from build123d import *

# Parameters (mm, degrees)
F0_W      = 40
F0_H      = 28
F1_DEPTH  = 1.5
F3_R      = 1.5
F4_DEPTH  = 1.501
F5_R      = 1.15
F6_DEPTH  = 1.501
F7_W      = 1.5
F7_H      = 28
F8_DEPTH  = 8
F9_R      = 3
F10_DEPTH = 1.501


with BuildPart() as f1:
    # F0 (on Front) → F1 (new body)
    with BuildSketch(Plane.XZ):
        with Locations((20, -14)):
            Rectangle(F0_W, F0_H)
    extrude(amount=F1_DEPTH)

    # F3 (on face) → F4 (cut, through all)
    with BuildSketch(Plane(origin=(0, 0, 0), x_dir=(-1, 0, 0), z_dir=(0, 1, 0))):
        with Locations((-38, -26)):
            Circle(F3_R)
        with Locations((-9, -24)):
            Circle(F3_R)
        with Locations((-9, -4)):
            Circle(F3_R)
    extrude(amount=-F4_DEPTH, mode=Mode.SUBTRACT)

    # F5 (on face) → F6 (cut, through all)
    with BuildSketch(Plane(origin=(0, 0, 0), x_dir=(-1, 0, 0), z_dir=(0, 1, 0))):
        with Locations((-20.5, -24)):
            Circle(F5_R)
        with Locations((-30.490284, -23.559283)):
            Circle(F5_R)
    extrude(amount=-F6_DEPTH, mode=Mode.SUBTRACT)

    # F7 (on face) → F8 (join)
    with BuildSketch(Plane.YZ.offset(40)):
        with Locations((-0.75, -14)):
            Rectangle(F7_W, F7_H)
    extrude(amount=F8_DEPTH)

    # F9 (on face) → F10 (cut, through all)
    with BuildSketch(Plane(origin=(0, 0, 0), x_dir=(-1, 0, 0), z_dir=(0, 1, 0))):
        with Locations((-38, -10)):
            Circle(F9_R)
    extrude(amount=-F10_DEPTH, mode=Mode.SUBTRACT)


solid = f1.part
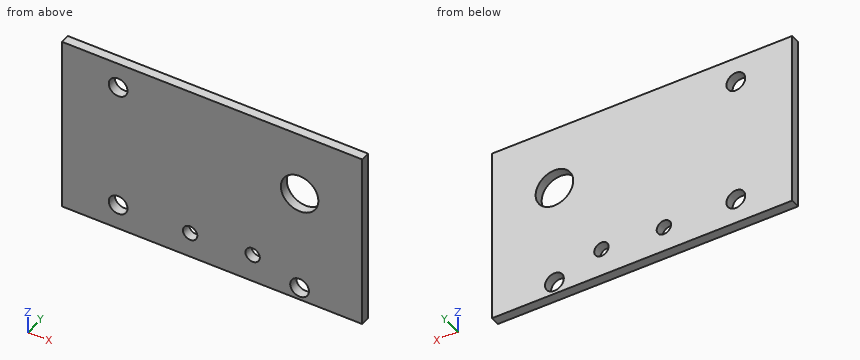
The model under review builds one solid part; all positions refer to its coordinate system, in mm. Round coordinates to 2 decimals unless told otherwise and drop trailing zeros. Loops run counter-clockwise (first coordinate to the right, second up) from the corner with the lowest first, then second, coordinate; pieces in that order, holes last. Notation, with made-up numbers: M 86,71 L 103,71 A20 cw 103,101 Z; hole C 88.5,-7 d8. An arc over 180 degrees is marked long. Answer as a JSON object with one key per item and string values.
Item 1: We need section B-B, the plane z = -10. State the section outline as (x, y) points, and give its area (3 significant figures).
Check sheet entries:
{"outline": "M 0,-1.5 L 35,-1.5 L 35,0 L 0,0 Z; M 41,-1.5 L 48,-1.5 L 48,0 L 41,0 Z", "area": "63.0 mm2"}
Item 2: We need section C-C, the plane x = 38. State the section outline as (y, z) points, and give its area (3 significant figures).
Check sheet entries:
{"outline": "M -1.5,-28 L 0,-28 L 0,-27.5 L -1.5,-27.5 Z; M -1.5,-24.5 L 0,-24.5 L 0,-13 L -1.5,-13 Z; M -1.5,-7 L 0,-7 L 0,0 L -1.5,0 Z", "area": "28.5 mm2"}
Item 3: Clearance check with flat-ended pins moving along their axes: P1, Ø2.5, axis at x = 9, z = -24, coming from the +Y side; P2, Ø5, axis at x = 30, z = -22.5, coming from the +Y side. State where each tip first meets the part, or that it passes through.
Check sheet entries:
{"P1": "through", "P2": "y = 0"}
Item 4: We need section D-D, the plane y = -1.1. State the section outline as (x, z) points.
Check sheet entries:
{"outline": "M 0,-28 L 48,-28 L 48,0 L 0,0 Z; hole C 9,-24 d3; hole C 9,-4 d3; hole C 20.5,-24 d2.3; hole C 30.49,-23.56 d2.3; hole C 38,-10 d6; hole C 38,-26 d3"}
Item 5: We need section A-A, the plane x = 9. State the section outline as (y, z) points, and give its area (3 significant figures).
Check sheet entries:
{"outline": "M -1.5,-28 L 0,-28 L 0,-25.5 L -1.5,-25.5 Z; M -1.5,-22.5 L 0,-22.5 L 0,-5.5 L -1.5,-5.5 Z; M -1.5,-2.5 L 0,-2.5 L 0,0 L -1.5,0 Z", "area": "33.0 mm2"}
Item 6: For line 1 along Z through (x, y) = (9, -0.9); line 2 along Z through (x, y) = (38, -1.1); line 3 along Z through (x, y) = (20.5, -0.55), list the stretches that pass through material, from the lowest coordinate up.
Check sheet entries:
{"line 1": "-28 to -25.5, -22.5 to -5.5, -2.5 to 0", "line 2": "-28 to -27.5, -24.5 to -13, -7 to 0", "line 3": "-28 to -25.15, -22.85 to 0"}
